```python
from build123d import *

# Parameters (mm, degrees)
SKETCH2_W           = 10
SKETCH2_H           = 3
BOSS_EXTRUDE1_DEPTH = 7
CUT_EXTRUDE2_DEPTH  = 13.56980509
LPATTERN2_COUNT     = 10
LPATTERN2_PITCH     = 2
FILLET2_START       = -1
FILLET2_DEPTH       = 9


with BuildPart() as part:
    # Sketch2 → Boss-Extrude1 (new body)
    with BuildSketch(Plane(origin=(0, 0, 0), x_dir=(0, 0, -1), z_dir=(1, 0, 0))):
        with Locations((5, -1.5)):
            Rectangle(SKETCH2_W, SKETCH2_H)
    extrude(amount=BOSS_EXTRUDE1_DEPTH)

    # Sketch1 → Cut-Extrude2 (cut, through all)
    with BuildSketch(Plane(origin=(0, 0, 0), x_dir=(0, 0, -1), z_dir=(1, 0, 0))):
        with BuildLine():
            ThreePointArc((0.10112359, -0.438202237), (0.045620517, -0.221237163), (0.080384758, 0))
            Line((0.080384758, 0), (0, 0))
            ThreePointArc((0, 0), (0.025608803, -0.224859501), (0.10112359, -0.438202237))
        make_face()
        with BuildLine():
            ThreePointArc((1.155, -0.195), (1.146082164, -0.095907769), (1.119615242, 0))
            Line((1.119615242, 0), (0.080384758, 0))
            ThreePointArc((0.080384758, 0), (0.045620517, -0.221237163), (0.10112359, -0.438202237))
            ThreePointArc((0.10112359, -0.438202237), (0.6, -0.75), (1.09887641, -0.438202237))
            ThreePointArc((1.09887641, -0.438202237), (1.140787115, -0.319797021), (1.155, -0.195))
        make_face()
        with BuildLine():
            Line((0.080384758, 0), (1.119615242, 0))
            ThreePointArc((1.119615242, 0), (0.6, 0.36), (0.080384758, 0))
        make_face()
        with BuildLine():
            ThreePointArc((1.09887641, -0.438202237), (1.174391197, -0.224859501), (1.2, 0))
            Line((1.2, 0), (1.119615242, 0))
            ThreePointArc((1.119615242, 0), (1.146082164, -0.095907769), (1.155, -0.195))
            ThreePointArc((1.155, -0.195), (1.140787115, -0.319797021), (1.09887641, -0.438202237))
        make_face()
    cut_extrude2 = extrude(amount=CUT_EXTRUDE2_DEPTH, mode=Mode.SUBTRACT)

    # LPattern2: Cut-Extrude2 ×10
    with Locations(*[(0, 0, -i * LPATTERN2_PITCH) for i in range(1, LPATTERN2_COUNT)]):
        add(cut_extrude2, mode=Mode.SUBTRACT)

    # Fillet2: read off the stored shape, not the designer's step
    # Fillet2 outline → Fillet2 (cut)
    with BuildSketch(Plane.YZ.offset(FILLET2_START)):
        with BuildLine():
            Line((0, -10), (0, -9.85))
            ThreePointArc((0, -9.85), (-0.043933983, -9.956066017), (-0.15, -10))
            Line((-0.15, -10), (0, -10))
        make_face()
        with BuildLine():
            ThreePointArc((-0.130434783, -9.191456891), (-0.037228588, -9.241268354), (0, -9.340175425))
            Line((0, -9.340175425), (0, -9.2))
            ThreePointArc((0, -9.2), (-0.065357129, -9.197861937), (-0.130434783, -9.191456891))
        make_face()
        with BuildLine():
            Line((0, -8), (0, -7.859824575))
            ThreePointArc((0, -7.859824575), (-0.037228588, -7.958731646), (-0.130434783, -8.008543109))
            ThreePointArc((-0.130434783, -8.008543109), (-0.065357129, -8.002138063), (0, -8))
        make_face()
        with BuildLine():
            ThreePointArc((-0.130434783, -7.191456891), (-0.037228588, -7.241268354), (0, -7.340175425))
            Line((0, -7.340175425), (0, -7.2))
            ThreePointArc((0, -7.2), (-0.065357129, -7.197861937), (-0.130434783, -7.191456891))
        make_face()
        with BuildLine():
            Line((0, -6), (0, -5.859824575))
            ThreePointArc((0, -5.859824575), (-0.037228588, -5.958731646), (-0.130434783, -6.008543109))
            ThreePointArc((-0.130434783, -6.008543109), (-0.065357129, -6.002138063), (0, -6))
        make_face()
        with BuildLine():
            ThreePointArc((-0.130434783, -5.191456891), (-0.037228588, -5.241268354), (0, -5.340175425))
            Line((0, -5.340175425), (0, -5.2))
            ThreePointArc((0, -5.2), (-0.065357129, -5.197861937), (-0.130434783, -5.191456891))
        make_face()
        with BuildLine():
            Line((0, -4), (0, -3.859824575))
            ThreePointArc((0, -3.859824575), (-0.037228588, -3.958731646), (-0.130434783, -4.008543109))
            ThreePointArc((-0.130434783, -4.008543109), (-0.065357129, -4.002138063), (0, -4))
        make_face()
        with BuildLine():
            ThreePointArc((-0.130434783, -3.191456891), (-0.037228588, -3.241268354), (0, -3.340175425))
            Line((0, -3.340175425), (0, -3.2))
            ThreePointArc((0, -3.2), (-0.065357129, -3.197861937), (-0.130434783, -3.191456891))
        make_face()
        with BuildLine():
            Line((0, -2), (0, -1.859824575))
            ThreePointArc((0, -1.859824575), (-0.037228588, -1.958731646), (-0.130434783, -2.008543109))
            ThreePointArc((-0.130434783, -2.008543109), (-0.065357129, -2.002138063), (0, -2))
        make_face()
        with BuildLine():
            ThreePointArc((-0.737701575, 0), (-0.601941305, -0.086210119), (-0.622233155, -0.245744681))
            ThreePointArc((-0.622233155, -0.245744681), (-0.537928158, -0.163622551), (-0.438202247, -0.101123596))
            ThreePointArc((-0.438202247, -0.101123596), (-0.224859507, -0.025608804), (0, 0))
            Line((0, 0), (-0.737701575, 0))
        make_face()
        with BuildLine():
            ThreePointArc((-0.130434783, -1.191456891), (-0.037228588, -1.241268354), (0, -1.340175425))
            Line((0, -1.340175425), (0, -1.2))
            ThreePointArc((0, -1.2), (-0.065357129, -1.197861937), (-0.130434783, -1.191456891))
        make_face()
    extrude(amount=FILLET2_DEPTH, mode=Mode.SUBTRACT)


solid = part.part
```
Here's how the part is built. I have some questions about the finished solid (model axes, mm). Give positions to 0.01 mm unless a question says otherwise; leave off trailing zeros. Loops run counter-clockwise (first coordinate to the right, second up) from the corner with the lowest first, then second, coordinate; pieces in that order, holes last. Notation, with made-up numbers: M 67,-29.75 L 89,-29.75 A21 cw 89,4.25 Z; hole C -12,39.25 d1. An arc over 180 degrees is marked long. Put each result on its own line as item: value. Start each with the question number.
(1) If we mould it in two halves opening along Z, with no side actions, what happens to faces 1 (the flat face through (3, -2, 0)), 2 (the cylindrical face through (3.45, -0.75, -8.59)), 3 (the flat face through (0, -2, -5))? For each: +Z half, -Z half, draft (parallel to the pull), parting line (faces both ways), or undercut.
(2) I want a section at B-B on z = -0.75. Please give me the cut outline in (x, y), then the cut area to 3 significant figures.
(3) I need wall thicknesses on line 1 along Z through (x, y) = (5.5, -0.4); line 2 along Z through (x, y) = (1, -0.55); line 3 along Y through (x, z) = (3.5, -2.5). Which ranges of each line are inside material? Lowest first, please. Write a range as [from, to].
Answer block:
1. face 1: +Z half
1. face 2: undercut
1. face 3: draft
2. outline: M 0,-3 L 7,-3 L 7,-0.73 L 0,-0.73 Z
2. area: 15.9 mm^2
3. line 1: [-10, -9.12], [-8.08, -7.12], [-6.08, -5.12], [-4.08, -3.12], [-2.08, -1.12]
3. line 2: [-10, -9.03], [-8.17, -7.03], [-6.17, -5.03], [-4.17, -3.03], [-2.17, -1.03]
3. line 3: [-3, -0.74]
